Design review of the part shown in the three views and the two pictorial views. Dimensions are in mm from the part's minimum x, y and z. A direction names the side the tool comes from. Give positions to 0.01 mm unless a question says otherwise; leave off trailing zeros. Order: outer loops, then holes, each group sorted by start corner. A loop starts at its lowest first (then second) coordinate and runs counter-clockwise, first axis right, second up. Notation, with made-up numbers: M -12.5,39 L 14.5,39 A12 ccw 14.5,57 Z; hole C -19.5,34.5 d6. An arc over 180 degrees is marked long. Answer as a JSON object with one key per item and string values.
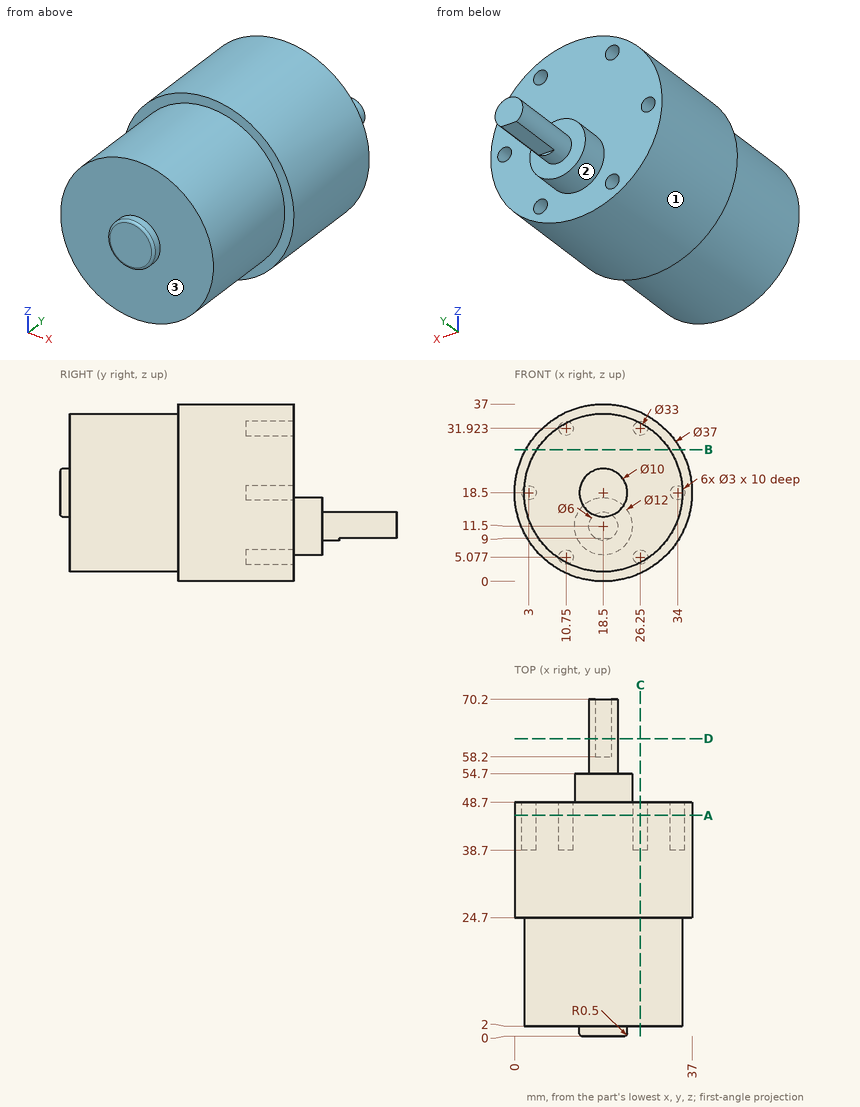
(1) We need section A-A (y = 46). Write out the cut boundary in (x, z).
Checked values:
{"outline": "C 18.5,18.5 d37; hole C 3,18.5 d3; hole C 10.75,5.08 d3; hole C 10.75,31.92 d3; hole C 26.25,5.08 d3; hole C 26.25,31.92 d3; hole C 34,18.5 d3"}
(2) We need section B-B (z = 27.5). Write out the cut boundary in (x, y).
Checked values:
{"outline": "M 2.34,24.7 L 4.67,24.7 L 4.67,2 L 32.33,2 L 32.33,24.7 L 34.66,24.7 L 34.66,48.7 L 2.34,48.7 Z"}
(3) We need section C-C (x = 26.25). Write out the cut boundary in (y, z), plus the area to 3 significant figures.
Checked values:
{"outline": "M 2,3.93 L 24.7,3.93 L 24.7,1.7 L 48.7,1.7 L 48.7,3.58 L 38.7,3.58 L 38.7,6.58 L 48.7,6.58 L 48.7,30.42 L 38.7,30.42 L 38.7,33.42 L 48.7,33.42 L 48.7,35.3 L 24.7,35.3 L 24.7,33.07 L 2,33.07 Z", "area": "1,410 mm^2"}
(4) To check wall thickness, follow L1, parallel to X at y = 43, z = 18.5; L2, parallel to Z at x = 10, y = 45 (1 decimal); L3, parallel to Y at x = 11, z = 5. State the ranges of each line that lie inside material, in increasing order. Write a range as from..to.
Checked values:
{"L1": "x = 0..1.5, 4.5..32.5, 35.5..37", "L2": "z = 2.1..3.8, 6.4..30.6, 33.2..34.9", "L3": "y = 2..38.7"}
(5) Insertion check: pin 1 (5 mm diameter, centred on x = 11, z = 14, fed in from -Y); pin 2 (5 mm diameter, centred on x = 29, y = 49, fed in from +Z); pin 3 (3.5 mm diameter, centred on x = 18.5, y = 65, fed in from -Z). Each pin has a flat end and moves straight along its axis. Give the tip position at first contact, or say it passes through.
Checked values:
{"pin 1": "stops at y = 2", "pin 2": "stops at z = 35.17", "pin 3": "stops at z = 9"}
(6) Tool access review of the marked faces 1, 2 and 3: name each direction out of +Z, -Z, +X, -X, +Y, -Y from which nothing blocks a thin tool from reaching the whole face with its end or side.
Checked values:
{"face 1": "+Y, -Y", "face 2": "+Y", "face 3": "-Y"}
(7) We need section D-D (y = 62). Write out the cut boundary in (x, z).
Checked values:
{"outline": "M 16.84,9 L 20.16,9 A3 ccw long Z"}
